Geometry: final body of the model. Coordinates: model frame, mm. A direction names the side the tool comes from. Give positions to 0.01 mm unless a question says otherwise; leave off trailing zeros. Loops run counter-clockwise (first coordinate to the right, second up) from the corner with the lowest first, then second, coordinate; pieces in that order, holes last. Notation, with made-up numbers: M 59,23 L 67,23 A15 cw 67,44 Z; hole C 62,55 d10. An arc over 180 degrees is marked long. Put each result on its own line as item: value.
```python
from build123d import *

# Parameters (mm, degrees)
BOSS_EXTRUDE1_DEPTH        = 10
BOSS_EXTRUDE2_DEPTH        = 2
F_3_5_3_5_DIAMETER_HOLE1_D = 3.5
SKETCH8_W                  = 12
SKETCH8_H                  = 8
CUT_EXTRUDE1_DEPTH         = 5
CHAMFER1_SIZE              = 1


with BuildPart() as part:
    # Sketch1 → Boss-Extrude1 (new body)
    with BuildSketch(Plane(origin=(0, 0, 0), x_dir=(1, 0, 0), z_dir=(0, 1, 0))):
        with BuildLine():
            Line((-23, 18.5), (23, 18.5))
            ThreePointArc((23, 18.5), (28.656854249, 16.156854249), (31, 10.5))
            Line((31, 10.5), (31, -10.5))
            ThreePointArc((31, -10.5), (28.656854249, -16.156854249), (23, -18.5))
            Line((23, -18.5), (-23, -18.5))
            ThreePointArc((-23, -18.5), (-28.656854249, -16.156854249), (-31, -10.5))
            Line((-31, -10.5), (-31, 10.5))
            ThreePointArc((-31, 10.5), (-28.656854249, 16.156854249), (-23, 18.5))
        make_face()
        with BuildLine():
            Line((-23, -15.5), (23, -15.5))
            ThreePointArc((23, -15.5), (26.535533906, -14.035533906), (28, -10.5))
            Line((28, -10.5), (28, 10.5))
            ThreePointArc((28, 10.5), (26.535533906, 14.035533906), (23, 15.5))
            Line((23, 15.5), (-23, 15.5))
            ThreePointArc((-23, 15.5), (-26.535533906, 14.035533906), (-28, 10.5))
            Line((-28, 10.5), (-28, -10.5))
            ThreePointArc((-28, -10.5), (-26.535533906, -14.035533906), (-23, -15.5))
        make_face(mode=Mode.SUBTRACT)
    extrude(amount=-BOSS_EXTRUDE1_DEPTH)

    # Sketch1_2 → Boss-Extrude2 (add)
    with BuildSketch(Plane(origin=(0, 0, 0), x_dir=(1, 0, 0), z_dir=(0, 1, 0))):
        with BuildLine():
            ThreePointArc((-28, 10.5), (-26.535533906, 14.035533906), (-23, 15.5))
            Line((-23, 15.5), (23, 15.5))
            ThreePointArc((23, 15.5), (26.535533906, 14.035533906), (28, 10.5))
            Line((28, 10.5), (28, -10.5))
            ThreePointArc((28, -10.5), (26.535533906, -14.035533906), (23, -15.5))
            Line((23, -15.5), (-23, -15.5))
            ThreePointArc((-23, -15.5), (-26.535533906, -14.035533906), (-28, -10.5))
            Line((-28, -10.5), (-28, 10.5))
        make_face()
    extrude(amount=-BOSS_EXTRUDE2_DEPTH)

    # Sketch4 → 3.3 _3.3_ Diameter Hole1 (revolve, cut)
    with BuildSketch(Plane(origin=(31, -5, 0), x_dir=(0, 0, -1), z_dir=(0, 1, 0))):
        Polygon((0, 0), (0, 10.991420021), (1.65, 10), (1.65, 0), align=None)
    f_3_3_3_3_diameter_hole1 = revolve(axis=Axis((37.35, -5, 0), (-1, 0, 0)), mode=Mode.SUBTRACT)

    # Mirror1: 3.3 _3.3_ Diameter Hole1 across plane
    add(f_3_3_3_3_diameter_hole1.mirror(Plane(origin=(0, 0, 0), x_dir=(0, 0, 1), z_dir=(1, 0, 0))), mode=Mode.SUBTRACT)

    # 3.5 _3.5_ Diameter Hole1 (through all)
    with Locations(Plane(origin=(0, -2, 0), x_dir=(-1, 0, 0), z_dir=(0, -1, 0))):
        with Locations((0, 0)):
            Hole(F_3_5_3_5_DIAMETER_HOLE1_D / 2)

    # Sketch8 → Cut-Extrude1 (cut)
    with BuildSketch(Plane.XY.offset(18.5)):
        with Locations((0, -6)):
            Rectangle(SKETCH8_W, SKETCH8_H)
    extrude(amount=-CUT_EXTRUDE1_DEPTH, mode=Mode.SUBTRACT)

    # Chamfer1
    chamfer1_edges = [part.edges().sort_by_distance(p)[0] for p in [
        (26.535533906, -10, -14.035533906),
        (28, -10, 0),
        (26.535533906, -10, 14.035533906),
        (-14.5, -10, 15.5),
        (-26.535533906, -10, 14.035533906),
        (-28, -10, 0),
        (-26.535533906, -10, -14.035533906),
        (0, -10, -15.5),
        (14.5, -10, 15.5),
    ]]
    chamfer(chamfer1_edges, length=CHAMFER1_SIZE)


solid = part.part
```
Item 1: Set-up query: faces 4 (the cylindrical face through (28.594, -4.93, -16.219)), 5 (the cylindrical face through (26.57, -5.45, -14)). Return all of +Z, -Z, +X, -X, +Y, -Y with unobstructed straight access to the full face (end or side cutting, diameter ignored); none if empty.
Output values:
face 4: -Z, +X, +Y, -Y
face 5: -Y
Item 2: Section B-B on y = -1. Output: boundary loops of the cut face in (x, z), then the cut area to 3 significant figures.
Output values:
outline: M -31,-10.5 A8 ccw -23,-18.5 L 23,-18.5 A8 ccw 31,-10.5 L 31,10.5 A8 ccw 23,18.5 L -23,18.5 A8 ccw -31,10.5 Z; hole C 0,0 d3.5
area: 2,230 mm²
Item 3: Section D-D on y = -5. Output: boundary loops of the cut face in (x, z), then the cut area to 3 significant figures.
Output values:
outline: M -31,-10.5 A8 ccw -23,-18.5 L 23,-18.5 A8 ccw 31,-10.5 L 31,-1.65 L 28,-1.65 L 28,-10.5 A5 cw 23,-15.5 L -23,-15.5 A5 cw -28,-10.5 L -28,-1.65 L -31,-1.65 Z; M -31,1.65 L -28,1.65 L -28,10.5 A5 cw -23,15.5 L -6,15.5 L -6,18.5 L -23,18.5 A8 ccw -31,10.5 Z; M 6,15.5 L 23,15.5 A5 cw 28,10.5 L 28,1.65 L 31,1.65 L 31,10.5 A8 ccw 23,18.5 L 6,18.5 Z
area: 469 mm²
Item 4: Line query: probe 1 along X at (y, z) = (-2.5, -6.5); probe 2 along Z at (x, y) = (17, -2.75); probe 3 along Z at (x, y) = (-29.25, -5). Output: solid intervals per line, ascending. Write a range as [from, to].
Output values:
probe 1: [-31, -28], [28, 31]
probe 2: [-18.5, -15.5], [15.5, 18.5]
probe 3: [-15.49, -1.65], [1.65, 15.49]
Item 5: Mould query, pull axis Z, two halves, no side actions, for faces 1 (the flat face through (0, -5, -15.5)), 2 (the flat face through (0, -5, -18.5)), 3 (the flat face through (0.3, -1.6, 18.5)). Classes: pulls with the +Z half, pulls with the -Z half, needs draft (parallel to the pull), parting line crosses it, or undercut.
Output values:
face 1: undercut
face 2: pulls with the -Z half
face 3: pulls with the +Z half
Item 6: Pin query (flat end, axial travel): pin 1 Ø4.5 at (x, z) = (0, 0) entering from -Y; pin 2 Ø2.5 at (y, z) = (-7.5, 17) entering from -X; pin 3 Ø0.9 at (y, z) = (-6.5, 17.5) entering from +X; pin 4 Ø3 at (y, z) = (-5, 0) entering from -X. Return the tip coordinate at first contact, or that it passes through.
Output values:
pin 1: y = -2
pin 2: x = -29.04
pin 3: x = 27.59
pin 4: through
Item 7: Section A-A on x = 0. Output: boundary loops of the cut face in (y, z), then the cut area to 3 significant figures.
Output values:
outline: M -10,-18.5 L 0,-18.5 L 0,-1.75 L -2,-1.75 L -2,-15.5 L -9,-15.5 L -10,-16.5 Z; M -2,1.75 L 0,1.75 L 0,18.5 L -2,18.5 Z
area: 90.5 mm²
Item 8: Section C-C on z = 0. Output: boundary loops of the cut face in (x, y), then the cut area to 3 significant figures.
Output values:
outline: M -31,-10 L -29,-10 L -28,-9 L -28,-6.65 L -31,-6.65 Z; M -31,-3.35 L -28,-3.35 L -28,-2 L -1.75,-2 L -1.75,0 L -31,0 Z; M 1.75,-2 L 28,-2 L 28,-3.35 L 31,-3.35 L 31,0 L 1.75,0 Z; M 28,-9 L 29,-10 L 31,-10 L 31,-6.65 L 28,-6.65 Z
area: 144 mm²
